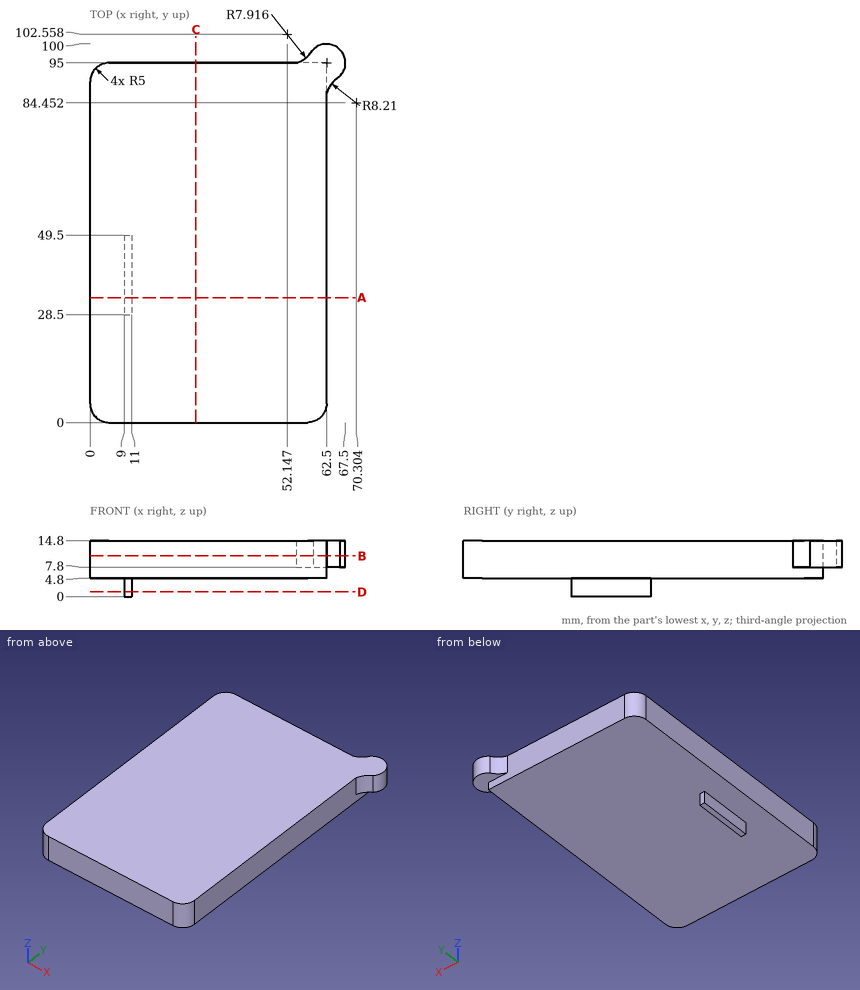
Answer from the drawing. Dimensions are ordinates in mm from the lowest x, y and z of the part. Round coordinates to 2 decimals unless told otherwise and drop trailing zeros. Loops run counter-clockwise (first coordinate to the right, second up) from the corner with the lowest first, then second, coordinate; pieces in that order, holes last.
Q1. Section B-B on z = 10.75 is taken. Write down the section's boundary in (x, y) (1 decimal).
Q2. Each of these flat-tipped pins is pushed along its axis until it touches: pin 1 (4 mm diameter, centred on x = 17, z = 2, fed in from -Y); pin 2 (1.4 mm diameter, centred on y = 39.5, z = 3, fed in from +X); pin 3 (1 mm diameter, centred on x = 10.5, z = 2.5, fed in from +Y); pin 4 (1.5 mm diameter, centred on y = 28.5, z = 2, fed in from -X). Where does it stop, or does it pass through?
Q3. Section A-A on y = 33 is taken. Write down the section's boundary in (x, z).
Q4. Consider probe 1 along Z at (x, y) = (22, 72.5); probe 2 along Y at (x, z) = (22.5, 5.75); probe 3 along X at (y, z) = (50.5, 8). Determine where each line is inside the solid, lowest interval first.
Q5. Section C-C on x = 28 is taken. Write down the section's boundary in (y, z).
Q6. Section D-D on z = 1.25 is taken. Write down the section's boundary in (x, y), and give its area (3 significant figures).
Output:
1. outline: (0, 5) arc R5 ccw to (5, 0) - (57.5, 0) arc R5 ccw to (62.5, 5) - (62.5, 87) arc R8.2 cw to (66, 91.5) arc R5 ccw to (59, 98.5) arc R7.9 cw to (54.5, 95) - (5, 95) arc R5 ccw to (0, 90) - close
2. pin 1: passes through
2. pin 2: stops at x = 11
2. pin 3: stops at y = 49.5
2. pin 4: stops at x = 9
3. outline: (0, 4.8) - (9, 4.8) - (9, 0) - (11, 0) - (11, 4.8) - (62.5, 4.8) - (62.5, 14.8) - (0, 14.8) - close
4. probe 1: z = 4.8 to 14.8
4. probe 2: y = 0 to 95
4. probe 3: x = 0 to 62.5
5. outline: (0, 4.8) - (95, 4.8) - (95, 14.8) - (0, 14.8) - close
6. outline: (9, 28.5) - (11, 28.5) - (11, 49.5) - (9, 49.5) - close
6. area: 42.0 mm2
